```python
from build123d import *

# Parameters (mm, degrees)
F1_DEPTH    = 79.375
F2_T1_DEPTH = 79.375
F2_T3_DEPTH = 92.075
F3_R        = 7.3025


# Not quite as in the source:
# - a fillet or chamfer that OpenCascade refuses, or shapes differently, is made with other operations: its cross-section is extruded or revolved along the edge and cut away or added


with BuildPart() as f1:
    # F0 (on Right) → F1 (new body)
    with BuildSketch(Plane.YZ):
        Polygon((0, 38.1), (0, 0), (38.1, 0), (38.1, 4.7625), (4.7625, 4.7625), (4.7625, 38.1), align=None)
    extrude(amount=F1_DEPTH)

    # F2: fillet of radius 2.54 on 5 edges, made by hand

    # F2_s2 → F2_t1 (join)
    with BuildSketch(Plane.YZ):
        with BuildLine():
            ThreePointArc((7.3025, 4.7625), (5.5064487758, 5.5064487758), (4.7625, 7.3025))
            Line((4.7625, 7.3025), (4.7625, 4.7625))
            Line((4.7625, 4.7625), (7.3025, 4.7625))
        make_face()
    extrude(amount=F2_T1_DEPTH)

    # F2_s4 → F2_t3 (cut)
    with BuildSketch(Plane.YZ.offset(-6.35)):
        with BuildLine():
            ThreePointArc((2.2225, 38.1), (4.0185512242, 37.3560512242), (4.7625, 35.56))
            Line((4.7625, 35.56), (4.7625, 38.1))
            Line((4.7625, 38.1), (2.2225, 38.1))
        make_face()
        with BuildLine():
            ThreePointArc((0, 35.56), (0.7439487758, 37.3560512242), (2.54, 38.1))
            Line((2.54, 38.1), (0, 38.1))
            Line((0, 38.1), (0, 35.56))
        make_face()
        with BuildLine():
            ThreePointArc((38.1, 2.2225), (37.3560512242, 4.0185512242), (35.56, 4.7625))
            Line((35.56, 4.7625), (38.1, 4.7625))
            Line((38.1, 4.7625), (38.1, 2.2225))
        make_face()
        with BuildLine():
            ThreePointArc((35.56, 0), (37.3560512242, 0.7439487758), (38.1, 2.54))
            Line((38.1, 2.54), (38.1, 0))
            Line((38.1, 0), (35.56, 0))
        make_face()
    extrude(amount=F2_T3_DEPTH, mode=Mode.SUBTRACT)

    # F3
    f3_edges = [f1.edges().sort_by_distance(p)[0] for p in [
        (39.6875, 0, 0),
    ]]
    fillet(f3_edges, radius=F3_R)


solid = f1.part
```
Geometry: final body of the model. Coordinates: model frame, mm. A direction names the side the tool comes from. Coordinates: 2 decimals unless noted, no trailing zeros. Order: outer loops, then holes, each group sorted by start corner. A loop starts at its lowest first (then second) coordinate and runs counter-clockwise, first axis right, second up. Notation, with made-up numbers: (53, 67) - (91, 67) arc R20 cw to (91, 99) - close; hole circle Ø9 at (-9.5, 61). An arc over 180 degrees is marked (long way). Return JSON: item names as keys, results as strings. Group by question number.
1. Cut plane A-A (x = 63). Output: boundary loops of the cut face in (y, z) (1 decimal), plus the area to 3 significant figures.
2. Set-up query: faces 1 (the face through (0, 10, 4)), 2 (the face through (39, 22, 4.762)). Return all of +Z, -Z, +X, -X, +Y, -Y with unobstructed straight access to the full face (end or side cutting, diameter ignored); none if empty.
3. Pin query (flat end, axial travel): pin 1 (3 mm diameter, centred on x = 44, z = 23, fed in from +Y); pin 2 (10 mm diameter, centred on y = 24, z = 12.5, fed in from +X); pin 3 (22.5 mm diameter, centred on x = 43, z = 17.5, fed in from +Y); pin 4 (10 mm diameter, centred on x = 59.5, z = 8, fed in from +Y). Return the tip coordinate at first contact, or that it passes through.
4. Cut plane B-B (y = 24). Output: boundary loops of the cut face in (x, z) (1 decimal), plus the area to 3 significant figures.
5. Material intervals for line 1 along Y through (x, z) = (76.5, 8); line 2 along Y through (x, z) = (11, 2), sorted ascending. Write a range as [from, to].
Resolved:
{
 "1": {"outline": "(0, 7.3) arc R7.3 ccw to (7.3, 0) - (35.6, 0) arc R2.5 ccw to (38.1, 2.4) arc R2.5 ccw to (35.6, 4.8) - (7.3, 4.8) arc R2.5 cw to (4.8, 7.3) - (4.8, 35.6) arc R2.5 ccw to (2.4, 38.1) arc R2.5 ccw to (0, 35.6) - close", "area": "325 mm²"},
 "2": {"face 1": "+Z, -Z, -X, +Y, -Y", "face 2": "+Z, +X, -X, +Y"},
 "3": {"pin 1": "stops at y = 4.76", "pin 2": "passes through", "pin 3": "stops at y = 4.99", "pin 4": "stops at y = 37.98"},
 "4": {"outline": "(0, 0) - (79.4, 0) - (79.4, 4.8) - (0, 4.8) - close", "area": "378 mm²"},
 "5": {"line 1": "y = [0, 4.76]", "line 2": "y = [2.28, 38.04]"}
}
